Here's the drawing with two shaded views (mm, measured from the low corner). I have some questions. Round coordinates to 2 decimals unless told otherwise and drop trailing zeros. Order: outer loops, then holes, each group sorted by start corner. A loop starts at its lowest first (then second) coordinate and runs counter-clockwise, first axis right, second up.
Q1. If we section it at D-D (y = 320): Please give me the cut outline in (x, z), plus the area to 3 significant figures.
Q2. If we section it at A-A (y = 130): Please give me the cut outline in (x, z), plus the area to 3 significant figures.
Q3. If we section it at B-B (z = 12.25): Please give me the cut outline in (x, y).
Q4. We'd pull the mould along X, two halves only. Please class the marked faces 1 and 2: pulls with the +X half, pulls with the -X half, needs draft (parallel to the pull), parting line crosses it, or undercut.
Q5. If we section it at C-C (x = 80): Please give me the cut outline in (y, z).
Q6. If I drill on line 1 (Y direction, x = 80, z = 6.5); line 2 (Y direction, x = 69.5, z = 8.5) (1 decimal); line 3 (X direction, y = 124, z = 3.5) (1 decimal), over which ranges is the centre line in solid material (lowest first)?
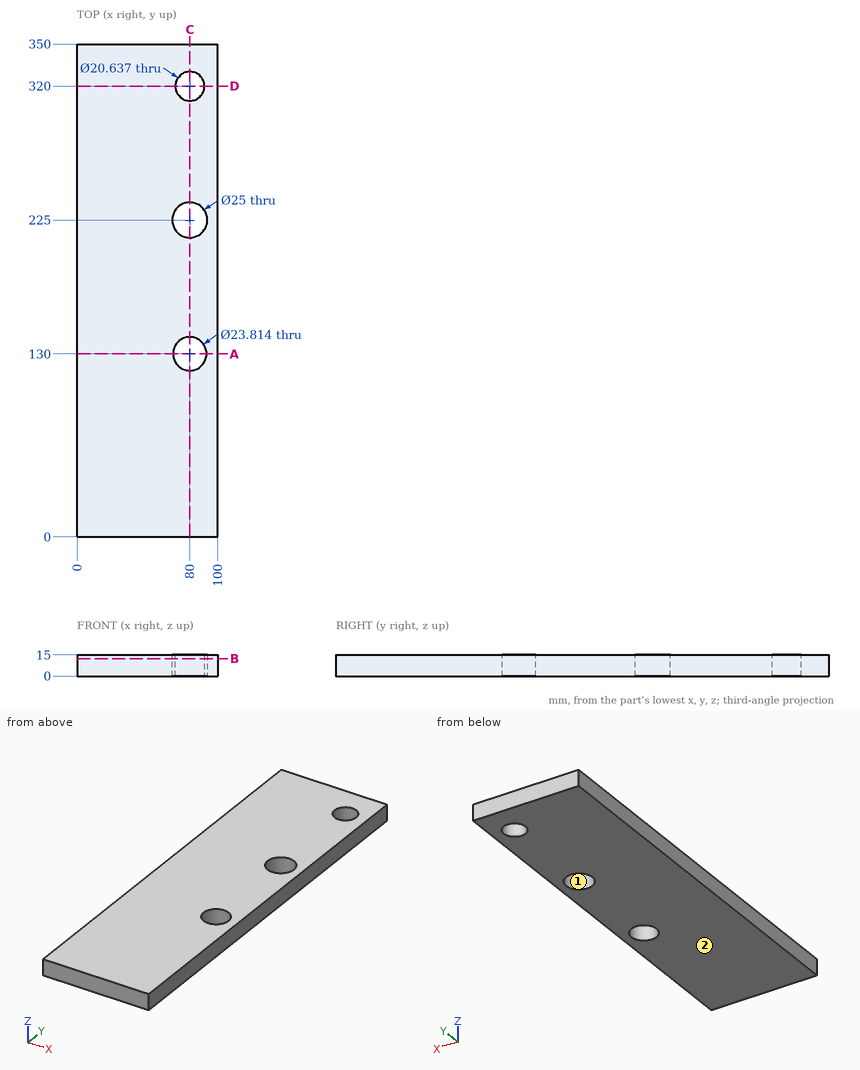
Solution:
1. outline: (0, 0) - (69.68, 0) - (69.68, 15) - (0, 15) - close; (90.32, 0) - (100, 0) - (100, 15) - (90.32, 15) - close
1. area: 1,190 mm2
2. outline: (0, 0) - (68.09, 0) - (68.09, 15) - (0, 15) - close; (91.91, 0) - (100, 0) - (100, 15) - (91.91, 15) - close
2. area: 1,140 mm2
3. outline: (0, 0) - (100, 0) - (100, 350) - (0, 350) - close; hole circle Ø25 at (80, 225); hole circle Ø23.81 at (80, 130); hole circle Ø20.64 at (80, 320)
4. face 1: undercut
4. face 2: needs draft
5. outline: (0, 0) - (118.09, 0) - (118.09, 15) - (0, 15) - close; (141.91, 0) - (212.5, 0) - (212.5, 15) - (141.91, 15) - close; (237.5, 0) - (309.68, 0) - (309.68, 15) - (237.5, 15) - close; (330.32, 0) - (350, 0) - (350, 15) - (330.32, 15) - close
6. line 1: y = 0 to 118.09, 141.91 to 212.5, 237.5 to 309.68, 330.32 to 350
6. line 2: y = 0 to 124.4, 135.6 to 218.2, 231.8 to 350
6. line 3: x = 0 to 69.7, 90.3 to 100
